from build123d import *

# Parameters (mm, degrees)
F0_W     = 5
F0_H     = 3
F0_W_2   = 15
F1_DEPTH = 3


with BuildPart() as f1:
    # F0 (on Right) → F1 (new body)
    with BuildSketch(Plane.YZ):
        with Locations((-14.5, 9.975)):
            Rectangle(F0_W, F0_H)
        with Locations((14.5, 9.975)):
            Rectangle(F0_W, F0_H)
        with Locations((0, -9.975)):
            Rectangle(F0_W_2, F0_H)
        Polygon((7.5, -8.475), (17, -8.475), (17, 8.475), (12, 8.475), (5, 8.475), (5, 5.475), (-5, 5.475), (-5, 8.475), (-12, 8.475), (-17, 8.475), (-17, -8.475), (-7.5, -8.475), align=None)
        Polygon((-17, 21.475), (-17, 11.475), (-12, 11.475), (-1.55, 11.475), (-1.55, 21.475), align=None)
        Polygon((12, 11.475), (17, 11.475), (17, 21.475), (1.55, 21.475), (1.55, 11.475), align=None)
    extrude(amount=F1_DEPTH)


solid = f1.part
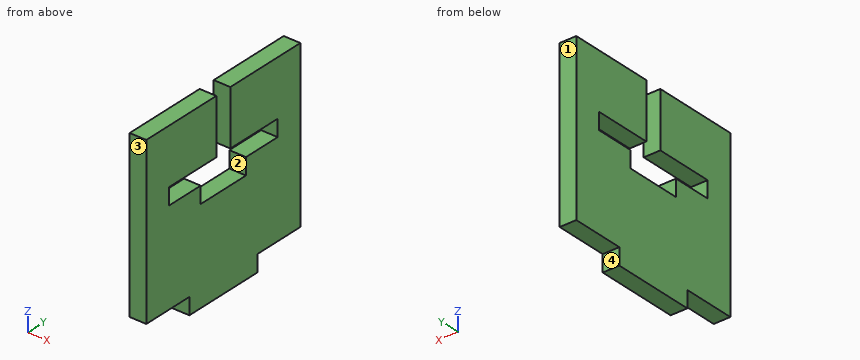
CAD build for the part. Positions are in the model's coordinates, mm. Face numbers are marked on the shaded views. A direction names the side the tool comes from. Give positions to 0.01 mm unless a question says otherwise; leave off trailing zeros. Loops run counter-clockwise (first coordinate to the right, second up) from the corner with the lowest first, then second, coordinate; pieces in that order, holes last. Notation, with made-up numbers: M -22,18 L -9,18 A23 cw -9,46 Z; hole C -14.75,28 d3. An arc over 180 degrees is marked long. Answer in a Markdown table with one row per item. Add a question column.
Item 1: Tool access for the marked faces 3 and 4: list every direction of +Z, -Z, +X, -X, +Y, -Y with a clear straight run to the whole face (end or side of a thin tool).
Item 2: Band-saw the part on D-D on y = -14. Give the cut face in (x, z) (3 decimals).
Item 3: Probe probe 1 along Y at (x, z) = (0.8, 15); probe 2 along Z at (x, y) = (1.2, -5.5) (3 decimals); probe 3 along Z at (x, y) = (2.15, 11) (3 decimals). List the from-to ranges inside material, lowest first.
Item 4: Drop flat-ended pins along their axis: P1, Ø1.5, axis at x = 1, z = -10.5, coming from the +Y side; P2, Ø0.9, axis at x = 1, y = 14, coming from the -Z side (3 decimals). Give the stop position or say it passes through.
Item 5: Band-saw the part on B-B on y = -9. Give the cut face in (x, z) (3 decimals).
Item 6: Band-saw the part on A-A on z = 12.5. Give the cut face in (x, y).
Item 7: Mould opens along Z. For the marked faces 1 and 2 say: +Z half, -Z half, draft (parallel to the pull), parting line (faces both ways), or undercut.
Item 8: Band-saw the part on C-C on x = 1.25. Give the cut face in (y, z) (3 decimals), then the cut area to 3 significant figures.
Reply:
| question | item | result |
|---|---|---|
| 1 | face 3 | +Z, -Z, +X, -X, -Y |
| 1 | face 4 | -Z, +X, -X, +Y |
| 2 | outline | M 0,-8.475 L 3,-8.475 L 3,21.475 L 0,21.475 Z |
| 3 | probe 1 | y = -17 to -1.55, 1.55 to 17 |
| 3 | probe 2 | z = -11.475 to 8.475, 11.475 to 21.475 |
| 3 | probe 3 | z = -8.475 to 8.475, 11.475 to 21.475 |
| 4 | P1 | stops at y = 7.5 |
| 4 | P2 | stops at z = -8.475 |
| 5 | outline | M 0,-8.475 L 3,-8.475 L 3,8.475 L 0,8.475 Z; M 0,11.475 L 3,11.475 L 3,21.475 L 0,21.475 Z |
| 6 | outline | M 0,-17 L 3,-17 L 3,-1.55 L 0,-1.55 Z; M 0,1.55 L 3,1.55 L 3,17 L 0,17 Z |
| 7 | face 1 | draft |
| 7 | face 2 | undercut |
| 8 | outline | M -17,-8.475 L -7.5,-8.475 L -7.5,-11.475 L 7.5,-11.475 L 7.5,-8.475 L 17,-8.475 L 17,21.475 L 1.55,21.475 L 1.55,11.475 L 12,11.475 L 12,8.475 L 5,8.475 L 5,5.475 L -5,5.475 L -5,8.475 L -12,8.475 L -12,11.475 L -1.55,11.475 L -1.55,21.475 L -17,21.475 Z |
| 8 | area | 930 mm^2 |
